```python
from build123d import *

# Parameters (mm, degrees)
F0_W     = 26
F0_H     = 46
F1_DEPTH = 170
F2_W     = 30
F2_H     = 50
F3_DEPTH = 1520
F4_W     = 60
F4_H     = 60
F4_R     = 6
F5_DEPTH = 5


with BuildPart() as f1:
    # F0 (on Front) → F1 (new body)
    with BuildSketch(Plane.XZ):
        Rectangle(F0_W, F0_H)
    extrude(amount=F1_DEPTH)

    # F2 (on face) → F3 (join)
    with BuildSketch(Plane.XZ.offset(170)):
        Rectangle(F2_W, F2_H)
    extrude(amount=F3_DEPTH)

    # F4 (on face) → F5 (join)
    with BuildSketch(Plane(origin=(0, 0, -25), x_dir=(1, 0, 0), z_dir=(0, 0, -1))):
        with Locations((-45, 1660)):
            Rectangle(F4_W, F4_H)
        with Locations((-50, 1645)):
            Circle(F4_R, mode=Mode.SUBTRACT)
        Polygon((15, 1690), (-15, 1690), (-15, 1630), (15, 1630), (15, 1645), align=None)
    extrude(amount=F5_DEPTH)


solid = f1.part
```
Can you work these out from the model? Positions are in its coordinate system, mm. A direction names the side the tool comes from. Give positions to 0.01 mm unless a question says otherwise; leave off trailing zeros. Write each loop counter-clockwise with the first axis right and the second up, starting at its lowest first coordinate (ties: lowest second). Pieces come first, ordered by that corner, then holes. Notation, with made-up numbers: (79, 69.25) - (87, 69.25) arc R15 ccw to (87, 98.25) - close; hole circle Ø8 at (33, 23.25). An arc over 180 degrees is marked (long way). Write item = value, one per line. Start each with the question number.
1. Imagine slicing it at B-B (y = -792). Please give me the cut outline in (x, z).
2. On a 3-axis mill with a long thin cutter (end or side, diameter ignored), from which of +Z, -Z, +X, -X, +Y, -Y can I reach the whole of each face in a straight line? I mean faces 1 (the face through (13, -84, 0)), 2 (the face through (0, -890, -25)), 3 (the face through (0, -84, 23)). Say none if no direction works.
3. Imagine slicing it at A-A (z = -1.5). Please give me the cut outline in (x, y), and give its area (3 significant figures).
4. Please list where these lines run through material, in increasing order: line 1 (X direction, y = -1645, z = -28.5); line 2 (Y direction, x = -50, z = -27.05); line 3 (Z direction, x = -11, y = -1105).
5. For pin 1 (4 mm diameter, centred on y = -1332.5, z = -20.5, fed in from -X); pin 2 (23 mm diameter, centred on y = -98.5, z = -11.5, fed in from -X); pin 3 (8 mm diameter, centred on x = 3, y = -85.5, fed in from +Z); pin 4 (9.5 mm diameter, centred on x = -50, y = -1645, fed in from -Z), each with a flat end and sliding along its axis, tell me the tip position at first contact or that it passes through.
Worked answers:
q1.outline = (-15, -25) - (15, -25) - (15, 25) - (-15, 25) - close
q2.face_1 = +Z, -Z, +X, +Y
q2.face_2 = -Z, +X, -X, +Y
q2.face_3 = +Z, +X, -X, +Y
q3.outline = (-15, -1690) - (15, -1690) - (15, -170) - (13, -170) - (13, 0) - (-13, 0) - (-13, -170) - (-15, -170) - close
q3.area = 50,000 mm2
q4.line_1 = -75 to -56, -44 to 15
q4.line_2 = -1690 to -1651, -1639 to -1630
q4.line_3 = -25 to 25
q5.pin_1 = -15
q5.pin_2 = -13
q5.pin_3 = 23
q5.pin_4 = through
